Check sheet for the modelled part. Datum: model origin and axes. Units: mm. Face numbers are marked on the shaded views. A direction names the side the tool comes from. Round coordinates to 2 decimals unless told otherwise and drop trailing zeros. Order: outer loops, then holes, each group sorted by start corner. A loop starts at its lowest first (then second) coordinate and runs counter-clockwise, first axis right, second up.
```python
from build123d import *

# Parameters (mm, degrees)
SALIENTE_EXTRUIR1_DEPTH      = 30.1625
SALIENTE_EXTRUIR1_DEPTH_BACK = 30.1625
CROQUIS1_R                   = 3.969
CROQUIS2_W                   = 53.975
CROQUIS2_H                   = 127
CORTAR_EXTRUIR1_DEPTH        = 138.343982508
CROQUIS3_R                   = 9.525
SALIENTE_EXTRUIR2_DEPTH      = 53.5
REDONDEO1_R                  = 6.35


with BuildPart() as part:
    # Croquis1 → Saliente-Extruir1 (new, two sides: drawn at the far end of the back side and taken through both)
    with BuildSketch(Plane.XY.offset(-SALIENTE_EXTRUIR1_DEPTH_BACK)):
        with BuildLine():
            Line((34.925, 95.25), (34.925, 107.95))
            Line((34.925, 107.95), (66.675, 107.95))
            Line((66.675, 107.95), (66.675, 95.25))
            ThreePointArc((66.675, 95.25), (50.749935163, 34.535310409), (7.075086505, -10.546712803))
            ThreePointArc((7.075086505, -10.546712803), (-10.546712803, -7.075086505), (-7.075086505, 10.546712803))
            ThreePointArc((-7.075086505, 10.546712803), (23.848499799, 47.977772084), (34.925, 95.25))
        make_face()
        Circle(CROQUIS1_R, mode=Mode.SUBTRACT)
    extrude(amount=SALIENTE_EXTRUIR1_DEPTH + SALIENTE_EXTRUIR1_DEPTH_BACK)

    # Croquis2 → Cortar-Extruir1 (cut, through all)
    with BuildSketch(Plane(origin=(66.675, 0, 0), x_dir=(0, 0, -1), z_dir=(1, 0, 0))):
        with Locations((0, 31.75)):
            Rectangle(CROQUIS2_W, CROQUIS2_H)
    extrude(amount=-CORTAR_EXTRUIR1_DEPTH, mode=Mode.SUBTRACT)

    # Croquis3 → Saliente-Extruir2 (add)
    with BuildSketch(Plane(origin=(0, 107.95, 0), x_dir=(1, 0, 0), z_dir=(0, 1, 0))):
        with Locations(Location((50.8, 0, 0), (0, 0, 270))):
            Circle(CROQUIS3_R)
    extrude(amount=SALIENTE_EXTRUIR2_DEPTH)

    # Redondeo1
    redondeo1_edges = [part.edges().sort_by_distance(p)[0] for p in [
        (34.925, 107.95, 0),
        (66.675, 107.95, 0),
        (50.8, 107.95, 30.1625),
        (50.8, 107.95, -30.1625),
    ]]
    fillet(redondeo1_edges, radius=REDONDEO1_R)


solid = part.part
```
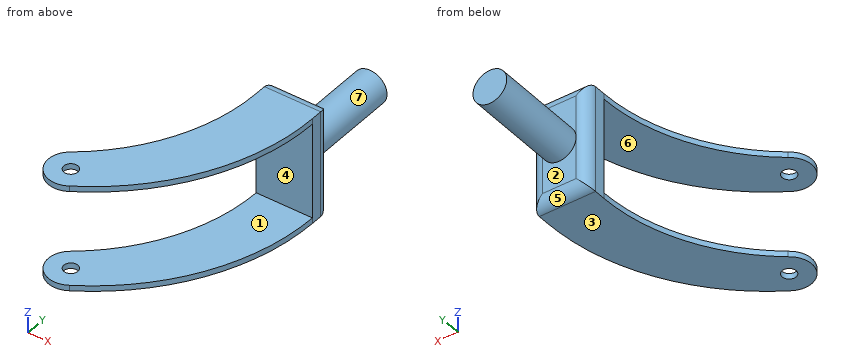
Item 1: Access from +Z, -Z, +X, -X, +Y, -Y to the whole of each face (thin tool, end or side, straight path). Record for the marked faces 5, 6 and 7.
Answer:
face 5: -Z, +X, -X, +Y
face 6: +X, -X, -Y
face 7: +Y
Item 2: Sectioned sample at C-C (x = 0). Record the cut outline in (y, z), and give its area (3 significant figures).
Answer:
outline: (-12.7, -30.16) - (-3.97, -30.16) - (-3.97, -26.99) - (-12.7, -26.99) - close; (-12.7, 26.99) - (-3.97, 26.99) - (-3.97, 30.16) - (-12.7, 30.16) - close; (3.97, -30.16) - (16.43, -30.16) - (16.43, -26.99) - (3.97, -26.99) - close; (3.97, 26.99) - (16.43, 26.99) - (16.43, 30.16) - (3.97, 30.16) - close
area: 135 mm2
Item 3: Sectioned sample at B-B (y = 31.5). Record the cut outline in (x, z), and give its area (3 significant figures).
Answer:
outline: (13.72, -30.16) - (48.98, -30.16) - (48.98, -26.99) - (13.72, -26.99) - close; (13.72, 26.99) - (48.98, 26.99) - (48.98, 30.16) - (13.72, 30.16) - close
area: 224 mm2
Item 4: Sectioned sample at A-A (x = 33). Record the cut outline in (y, z), and give its area (3 significant figures).
Answer:
outline: (10.41, -30.16) - (75.1, -30.16) - (75.1, -26.99) - (10.41, -26.99) - close; (10.41, 26.99) - (75.1, 26.99) - (75.1, 30.16) - (10.41, 30.16) - close
area: 411 mm2
Item 5: Sectioned sample at D-D (z = -16). Record the cut outline in (x, y) (3 decimals).
Answer:
outline: (34.925, 95.25) - (66.675, 95.25) - (66.675, 101.6) arc R6.35 ccw to (60.325, 107.95) - (41.275, 107.95) arc R6.35 ccw to (34.925, 101.6) - close
Item 6: Scan lines: line 1 along Z through (x, y) = (31, 19.5); line 2 along Y through (x, z) = (53, 23.5); line 3 along X through (y, z) = (0, 29.1). Record each from-to range of solid material in increasing order.
Answer:
line 1: z = -30.16 to -26.99, 26.99 to 30.16
line 2: y = 95.25 to 107.95
line 3: x = -12.7 to -3.97, 3.97 to 21.9
Item 7: Go/stop test with flat-tipped pins: P1, Ø12, axis at x = 17.5, z = 20, coming from the -Y side; P2, Ø1.9, axis at y = 98, z = 1, coming from the -X side (3 decimals). Record where each tip stops, or that it passes through.
Answer:
P1: passes through
P2: stops at x = 34.925
Item 8: Release check for a two-part mould opening along Z. For the marked faces 1, 2, 3 and 4 record: released by +Z, released by -Z, zero draft, split by the parting line, or undercut.
Answer:
face 1: undercut
face 2: zero draft
face 3: released by -Z
face 4: undercut
